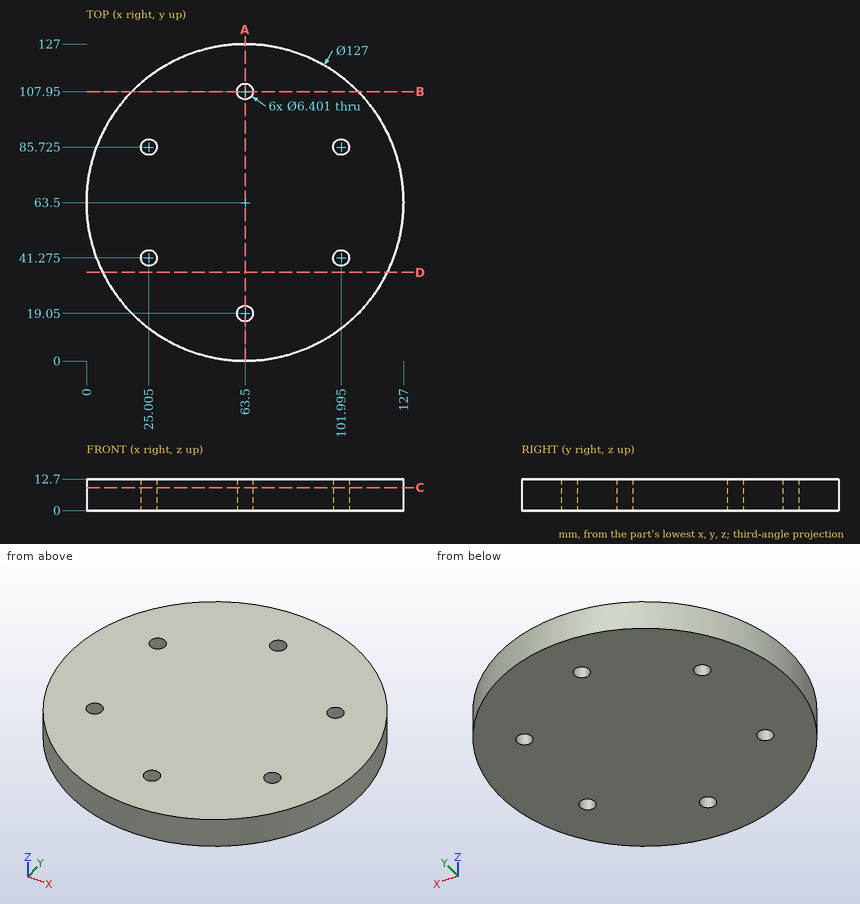
Geometry: see drawing. Coordinates: mm, zero at the bounding-box minimum. Round coordinates to 2 decimals unless told otherwise and drop trailing zeros. Order: outer loops, then holes, each group sorted by start corner. A loop starts at its lowest first (then second) coordinate and runs counter-clockwise, first axis right, second up. Notation, with made-up numbers: (18.25, 23) - (40.25, 23) arc R20 ccw to (40.25, 28) - close; hole circle Ø8 at (42.25, 7). An arc over 180 degrees is marked (long way). Use a Markdown table: item, result. Add a question column.
1. First-contact query: pin 1 (5 mm diameter, centred on x = 15, z = 5, fed in from +Y) (1 decimal); pin 2 (1 mm diameter, centred on x = 98, z = 7, fed in from -Y); pin 3 (3 mm diameter, centred on x = 29, z = 2, fed in from -Y). Flat tips, straight axial feed; report the tip coordinate or a pass-through.
2. Section query C-C (z = 9.25). Give the number of separate pieces and of enclosed holes in the cut face, then the cut area to 3 significant figures.
3. Section query D-D (y = 35.5). Return the cut outline in (x, z), then the cut area to 3 significant figures.
4. Section query A-A (x = 63.5). Return the cut outline in (y, z), then the cut area to 3 significant figures.
5. Line query: probe 1 along X at (y, z) = (38.5, 7); probe 2 along Y at (x, z) = (62.5, 6.5); probe 3 along Y at (x, z) = (22.5, 7). Output: solid intervals per line, ascending.
6. Section query B-B (y = 107.95). Return the cut outline in (x, z), then the cut area to 3 significant figures.
Derived:
| question | item | result |
|---|---|---|
| 1 | pin 1 | y = 107.3 |
| 1 | pin 2 | y = 9.87 |
| 1 | pin 3 | y = 9.25 |
| 2 | separate pieces | 1 |
| 2 | enclosed holes | 6 |
| 2 | area | 12,500 mm2 |
| 3 | outline | (6.51, 0) - (120.49, 0) - (120.49, 12.7) - (6.51, 12.7) - close |
| 3 | area | 1,450 mm2 |
| 4 | outline | (0, 0) - (15.85, 0) - (15.85, 12.7) - (0, 12.7) - close; (22.25, 0) - (104.75, 0) - (104.75, 12.7) - (22.25, 12.7) - close; (111.15, 0) - (127, 0) - (127, 12.7) - (111.15, 12.7) - close |
| 4 | area | 1,450 mm2 |
| 5 | probe 1 | 5.13 to 23.41, 26.6 to 100.4, 103.59 to 121.87 |
| 5 | probe 2 | 0.01 to 16.01, 22.09 to 104.91, 110.99 to 126.99 |
| 5 | probe 3 | 15.01 to 39.28, 43.27 to 83.73, 87.72 to 111.99 |
| 6 | outline | (18.15, 0) - (60.3, 0) - (60.3, 12.7) - (18.15, 12.7) - close; (66.7, 0) - (108.85, 0) - (108.85, 12.7) - (66.7, 12.7) - close |
| 6 | area | 1,070 mm2 |
